For this review, take the finished solid that the model builds, in its own axes (mm). Coordinates: 2 decimals unless noted, no trailing zeros. Write each loop counter-clockwise with the first axis right and the second up, starting at its lowest first coordinate (ties: lowest second). Pieces come first, ordered by that corner, then holes.
```python
from build123d import *

# Parameters (mm, degrees)
F0_R     = 1.27
F1_DEPTH = 1.6


with BuildPart() as f1:
    # F0 (on Top) → F1 (new body)
    with BuildSketch(Plane.XY):
        with BuildLine():
            Line((22.86, 11.43), (-22.86, 11.43))
            ThreePointArc((-22.86, 11.43), (-24.656051, 10.686051), (-25.4, 8.89))
            Line((-25.4, 8.89), (-25.4, -8.89))
            ThreePointArc((-25.4, -8.89), (-24.656051, -10.686051), (-22.86, -11.43))
            Line((-22.86, -11.43), (22.86, -11.43))
            ThreePointArc((22.86, -11.43), (24.656051, -10.686051), (25.4, -8.89))
            Line((25.4, -8.89), (25.4, 8.89))
            ThreePointArc((25.4, 8.89), (24.656051, 10.686051), (22.86, 11.43))
        make_face()
        with Locations((-22.86, -8.89)):
            Circle(F0_R, mode=Mode.SUBTRACT)
        with Locations((22.86, -8.89)):
            Circle(F0_R, mode=Mode.SUBTRACT)
        with Locations((-22.86, 8.89)):
            Circle(F0_R, mode=Mode.SUBTRACT)
        with Locations((22.86, 8.89)):
            Circle(F0_R, mode=Mode.SUBTRACT)
    extrude(amount=-F1_DEPTH)


solid = f1.part
```
Q1. Add section A-A (z = -1.05). State the section outline as (x, y) points.
Ans:
outline: (-25.4, -8.89) arc R2.54 ccw to (-22.86, -11.43) - (22.86, -11.43) arc R2.54 ccw to (25.4, -8.89) - (25.4, 8.89) arc R2.54 ccw to (22.86, 11.43) - (-22.86, 11.43) arc R2.54 ccw to (-25.4, 8.89) - close; hole circle Ø2.54 at (-22.86, -8.89); hole circle Ø2.54 at (-22.86, 8.89); hole circle Ø2.54 at (22.86, -8.89); hole circle Ø2.54 at (22.86, 8.89)
Q2. For probe 1 along Y at (x, z) = (22.86, -1.05); probe 2 along X at (y, z) = (-10, -1); probe 3 along X at (y, z) = (8.5, -1.45), list the stretches that pass through material, from the lowest coordinate up.
Ans:
probe 1: y = -11.43 to -10.16, -7.62 to 7.62, 10.16 to 11.43
probe 2: x = -25.14 to -23.48, -22.24 to 22.24, 23.48 to 25.14
probe 3: x = -25.4 to -24.07, -21.65 to 21.65, 24.07 to 25.4
Q3. Add section B-B (y = -9.5). State the section outline as (x, z) points.
Ans:
outline: (-25.33, -1.6) - (-23.97, -1.6) - (-23.97, 0) - (-25.33, 0) - close; (-21.75, -1.6) - (21.75, -1.6) - (21.75, 0) - (-21.75, 0) - close; (23.97, -1.6) - (25.33, -1.6) - (25.33, 0) - (23.97, 0) - close
Q4. Draft analysis for pull direction Y (two halves, no side actions). For faces 1 (the cylindrical face through (-21.65, -8.51, -0.79)), 2 (the flat face through (0, -11.43, -1)), 3 (the cylindrical face through (-24.636, 10.706, -0.789)), state which applies: +Y half, -Y half, draft (parallel to the pull), parting line (faces both ways), or undercut.
Ans:
face 1: undercut
face 2: -Y half
face 3: +Y half
